Build history of the part. All positions in model axes, mm. A direction names the side the tool comes from. Round coordinates to 2 decimals unless told otherwise and drop trailing zeros. Order: outer loops, then holes, each group sorted by start corner. A loop starts at its lowest first (then second) coordinate and runs counter-clockwise, first axis right, second up. Notation, with made-up numbers: (-11, 56) -> (34, 56) arc R16 cw to (34, 65) -> close; hole circle Ø9 at (45.25, 24). An arc over 180 degrees is marked (long way). Use a Markdown table: item, result. Add a question column.
Item 1: Probe L1, parallel to Z at x = 94, y = 1.5; L2, parallel to Z at x = 107, y = 0.25; L3, parallel to X at y = 0.4, z = 11. List the from-to ranges inside material, lowest first.
Item 2: Two-plate mould, pull along Z, no slides. Class faces 1 (the face through (56, 2, 0)), 2 (the face through (63.8, 1.83, 4.75)), 3 (the face through (45, 0, 6)): released by +Z, released by -Z, zero draft, split by the parting line, or undercut.
Item 3: Slice it at A-A, the plane x = 46. Give the cut face in (y, z).
Item 4: Slice it at B-B, the plane z = 23. Give the cut face in (x, y), plus the area to 3 significant figures.
Item 5: Slice it at D-D, the plane x = 89. Give the cut face in (y, z), plus the area to 3 significant figures.
Item 6: 3-axis set-ups, long thin cutter, end or side, ignore diameter. For faces 4 (the face through (59, 2, 9)), 5 (the face through (0.57, 1.77, 0.6)): which of +Z, -Z, +X, -X, +Y, -Y reach the whole face in a straight line?
Item 7: Slice it at C-C, the plane y = 2.3. State how many separate pieces and enclosed holes the cut face has, plus the area to 3 significant figures.
Item 8: Pin check, flat tips, straight feed: pin 1 (6 mm diameter, centred on x = 62, z = 34, fed in from +Y); pin 2 (3 mm diameter, centred on x = 86, z = 34, fed in from +Y). Stop position of each tip, or through.
from build123d import *

# Parameters (mm, degrees)
BOSS_EXTRUDE1_DEPTH = 3.6
SKETCH2_R           = 1.95
SKETCH2_W           = 100
SKETCH2_H           = 20
CUT_EXTRUDE1_DEPTH  = 3.6


with BuildPart() as part:
    # Sketch1 → Boss-Extrude1 (new body)
    with BuildSketch(Plane(origin=(0, 0, 0), x_dir=(1, 0, 0), z_dir=(0, 1, 0))):
        with BuildLine():
            Line((2, 0), (112, 0))
            ThreePointArc((112, 0), (113.414213562, -0.585786438), (114, -2))
            Line((114, -2), (114, -36))
            ThreePointArc((114, -36), (113.414213562, -37.414213562), (112, -38))
            Line((112, -38), (2, -38))
            ThreePointArc((2, -38), (0.585786438, -37.414213562), (0, -36))
            Line((0, -36), (0, -2))
            ThreePointArc((0, -2), (0.585786438, -0.585786438), (2, 0))
        make_face()
    extrude(amount=BOSS_EXTRUDE1_DEPTH)

    # Sketch2 → Cut-Extrude1 (cut)
    with BuildSketch(Plane(origin=(0, 3.6, 0), x_dir=(1, 0, 0), z_dir=(0, 1, 0))):
        with Locations((110, -4)):
            Circle(SKETCH2_R)
        with Locations((102, -4)):
            Circle(SKETCH2_R)
        with Locations((18, -4)):
            Circle(SKETCH2_R)
        with Locations((46, -4)):
            Circle(SKETCH2_R)
        with Locations((54, -4)):
            Circle(SKETCH2_R)
        with Locations((62, -4)):
            Circle(SKETCH2_R)
        with Locations((70, -4)):
            Circle(SKETCH2_R)
        with Locations((78, -4)):
            Circle(SKETCH2_R)
        with Locations((86, -4)):
            Circle(SKETCH2_R)
        with Locations((94, -4)):
            Circle(SKETCH2_R)
        with Locations((110, -34)):
            Circle(SKETCH2_R)
        with Locations((102, -34)):
            Circle(SKETCH2_R)
        with Locations((18, -34)):
            Circle(SKETCH2_R)
        with Locations((46, -34)):
            Circle(SKETCH2_R)
        with Locations((54, -34)):
            Circle(SKETCH2_R)
        with Locations((62, -34)):
            Circle(SKETCH2_R)
        with Locations((70, -34)):
            Circle(SKETCH2_R)
        with Locations((78, -34)):
            Circle(SKETCH2_R)
        with Locations((86, -34)):
            Circle(SKETCH2_R)
        with Locations((94, -34)):
            Circle(SKETCH2_R)
        with Locations((60, -19)):
            Rectangle(SKETCH2_W, SKETCH2_H)
    extrude(amount=-CUT_EXTRUDE1_DEPTH, mode=Mode.SUBTRACT)


solid = part.part
Check sheet entries:
| question | item | result |
|---|---|---|
| 1 | L1 | 0 to 2.05, 5.95 to 9, 29 to 32.05, 35.95 to 38 |
| 1 | L2 | 0 to 9, 29 to 38 |
| 1 | L3 | 0 to 10, 110 to 114 |
| 2 | face 1 | released by -Z |
| 2 | face 2 | undercut |
| 2 | face 3 | zero draft |
| 3 | outline | (0, 0) -> (3.6, 0) -> (3.6, 2.05) -> (0, 2.05) -> close; (0, 5.95) -> (3.6, 5.95) -> (3.6, 9) -> (0, 9) -> close; (0, 29) -> (3.6, 29) -> (3.6, 32.05) -> (0, 32.05) -> close; (0, 35.95) -> (3.6, 35.95) -> (3.6, 38) -> (0, 38) -> close |
| 4 | outline | (0, 0) -> (10, 0) -> (10, 3.6) -> (0, 3.6) -> close; (110, 0) -> (114, 0) -> (114, 3.6) -> (110, 3.6) -> close |
| 4 | area | 50.4 mm2 |
| 5 | outline | (0, 0) -> (3.6, 0) -> (3.6, 9) -> (0, 9) -> close; (0, 29) -> (3.6, 29) -> (3.6, 38) -> (0, 38) -> close |
| 5 | area | 64.8 mm2 |
| 6 | face 4 | +Y, -Y |
| 6 | face 5 | -Z, -X, +Y, -Y |
| 7 | separate pieces | 1 |
| 7 | enclosed holes | 21 |
| 7 | area | 2,090 mm2 |
| 8 | pin 1 | y = 3.6 |
| 8 | pin 2 | through |
